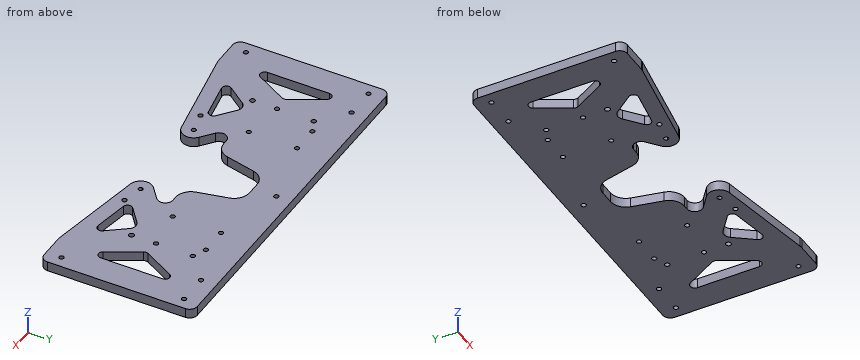
```python
from build123d import *

# Parameters (mm, degrees)
SKETCH1_W           = 233.2
SKETCH1_H           = 100
SKETCH1_R           = 1.55
BOSS_EXTRUDE1_DEPTH = 6.35
FILLET1_R           = 5
SKETCH2_R           = 1.55
CUT_EXTRUDE1_DEPTH  = 6.35
SKETCH3_W           = 10
SKETCH3_H           = 12.7
BOSS_EXTRUDE2_DEPTH = 6.35
FILLET2_R           = 5
FILLET3_R           = 10
FILLET4_R           = 2
FILLET5_R           = 20
FILLET6_R           = 5
CUT_EXTRUDE2_DEPTH  = 10
SKETCH5_W           = 120
SKETCH5_H           = 40
CUT_EXTRUDE4_DEPTH  = 10
SKETCH6_R           = 1.5
CUT_EXTRUDE5_DEPTH  = 10
FILLET7_R           = 10
SKETCH7_W           = 25
SKETCH7_H           = 35
CUT_EXTRUDE6_DEPTH  = 10
FILLET9_R           = 10
SKETCH8_R           = 1.5
CUT_EXTRUDE7_DEPTH  = 10
BOSS_EXTRUDE3_DEPTH = 6.35
FILLET10_R          = 5
BOSS_EXTRUDE4_DEPTH = 6.35
FILLET11_R          = 3
FILLET12_R          = 3
CUT_EXTRUDE8_DEPTH  = 10
FILLET13_R          = 3
CUT_EXTRUDE9_DEPTH  = 10
SKETCH13_R          = 1.55
CUT_EXTRUDE10_DEPTH = 10


with BuildPart() as part:
    # Sketch1 → Boss-Extrude1 (new body)
    with BuildSketch(Plane.XY):
        with Locations((116.6, -50)):
            Rectangle(SKETCH1_W, SKETCH1_H)
        with Locations((7.5, -10)):
            Circle(SKETCH1_R, mode=Mode.SUBTRACT)
        with Locations((225.7, -10)):
            Circle(SKETCH1_R, mode=Mode.SUBTRACT)
        with Locations((7.5, -90)):
            Circle(SKETCH1_R, mode=Mode.SUBTRACT)
        with Locations((225.7, -90)):
            Circle(SKETCH1_R, mode=Mode.SUBTRACT)
        with Locations((27.5, -10)):
            Circle(SKETCH1_R, mode=Mode.SUBTRACT)
        with Locations((205.7, -10)):
            Circle(SKETCH1_R, mode=Mode.SUBTRACT)
        with Locations((116.6, -10)):
            Circle(SKETCH1_R, mode=Mode.SUBTRACT)
    extrude(amount=BOSS_EXTRUDE1_DEPTH)

    # Fillet1
    fillet1_edges = [part.edges().sort_by_distance(p)[0] for p in [
        (233.2, -100, 3.175),
        (0, -100, 3.175),
        (0, 0, 3.175),
        (233.2, 0, 3.175),
    ]]
    fillet(fillet1_edges, radius=FILLET1_R)

    # Sketch2 → Cut-Extrude1 (cut)
    with BuildSketch(Plane.XY.offset(6.35)):
        with Locations((45, -25)):
            Circle(SKETCH2_R)
        with Locations((45, -49)):
            Circle(SKETCH2_R)
        with Locations(Location((188.2, -49, 0), (0, 0, 180))):
            Circle(SKETCH2_R)
        with Locations(Location((188.2, -25, 0), (0, 0, 180))):
            Circle(SKETCH2_R)
    extrude(amount=-CUT_EXTRUDE1_DEPTH, mode=Mode.SUBTRACT)

    # Sketch3 → Boss-Extrude2 (add)
    with BuildSketch(Plane.XY.offset(6.35)):
        with Locations((125.723568259, 6.35)):
            Rectangle(SKETCH3_W, SKETCH3_H)
        Polygon((120.723568259, 16.7), (120.723568259, 12.7), (130.723568259, 12.7), (130.723568259, 24.7), (85.723568259, 24.7), (85.723568259, 12.7), (95.723568259, 12.7), (95.723568259, 16.7), align=None)
        Polygon((130.723568259, 12.7), (130.723568259, 0), (152.313568259, 0), (130.723568259, 24.7), align=None)
    extrude(amount=-BOSS_EXTRUDE2_DEPTH)

    # Fillet2
    fillet2_edges = [part.edges().sort_by_distance(p)[0] for p in [
        (85.723568259, 12.7, 3.175),
    ]]
    fillet(fillet2_edges, radius=FILLET2_R)

    # Fillet3
    fillet3_edges = [part.edges().sort_by_distance(p)[0] for p in [
        (120.723568259, 0, 3.175),
    ]]
    fillet(fillet3_edges, radius=FILLET3_R)

    # Fillet4
    fillet4_edges = [part.edges().sort_by_distance(p)[0] for p in [
        (85.723568259, 24.7, 3.175),
    ]]
    fillet(fillet4_edges, radius=FILLET4_R)

    # Fillet5
    fillet5_edges = [part.edges().sort_by_distance(p)[0] for p in [
        (130.723568259, 24.7, 3.175),
        (152.313568259, 0, 3.175),
    ]]
    fillet(fillet5_edges, radius=FILLET5_R)

    # Fillet6
    fillet6_edges = [part.edges().sort_by_distance(p)[0] for p in [
        (120.723568259, 16.7, 3.175),
    ]]
    fillet(fillet6_edges, radius=FILLET6_R)

    # Sketch4 → Cut-Extrude2 (cut)
    with BuildSketch(Plane(origin=(0, 0, 0), x_dir=(-1, 0, 0), z_dir=(0, 0, -1))):
        with BuildLine():
            Line((-110.723568259, 0), (-161.395157905, 0))
            ThreePointArc((-161.395157905, 0), (-153.126132222, 1.789475179), (-146.33682816, 6.837678575))
            Line((-146.33682816, 6.837678575), (-136.700308357, 17.862321425))
            ThreePointArc((-136.700308357, 17.862321425), (-129.911004296, 22.910524821), (-121.641978613, 24.7))
            Line((-121.641978613, 24.7), (-87.723568259, 24.7))
            ThreePointArc((-87.723568259, 24.7), (-86.309354696, 24.114213562), (-85.723568259, 22.7))
            Line((-85.723568259, 22.7), (-85.723568259, 17.7))
            ThreePointArc((-85.723568259, 17.7), (-87.188034353, 14.164466094), (-90.723568259, 12.7))
            Line((-90.723568259, 12.7), (-95.723568259, 12.7))
            Line((-95.723568259, 12.7), (-95.723568259, 16.7))
            Line((-95.723568259, 16.7), (-115.723568259, 16.7))
            ThreePointArc((-115.723568259, 16.7), (-119.259102165, 15.235533906), (-120.723568259, 11.7))
            Line((-120.723568259, 11.7), (-120.723568259, 10))
            ThreePointArc((-120.723568259, 10), (-117.794636071, 2.928932188), (-110.723568259, 0))
        make_face()
    extrude(amount=-CUT_EXTRUDE2_DEPTH, mode=Mode.SUBTRACT)

    # Sketch5 → Cut-Extrude4 (cut)
    with BuildSketch(Plane.XY.offset(6.35)):
        Polygon((56.6, -100), (56.6, -60), (26.6, -100), align=None)
        with Locations((116.6, -80)):
            Rectangle(SKETCH5_W, SKETCH5_H)
        Polygon((206.6, -100), (176.6, -60), (176.6, -100), align=None)
    extrude(amount=-CUT_EXTRUDE4_DEPTH, mode=Mode.SUBTRACT)

    # Sketch6 → Cut-Extrude5 (cut)
    with BuildSketch(Plane.XY.offset(6.35)):
        with Locations((71.6, -21.25)):
            Circle(SKETCH6_R)
        with Locations((161.6, -21.25)):
            Circle(SKETCH6_R)
        with Locations((161.6, -52.75)):
            Circle(SKETCH6_R)
        with Locations((71.6, -52.75)):
            Circle(SKETCH6_R)
    extrude(amount=-CUT_EXTRUDE5_DEPTH, mode=Mode.SUBTRACT)

    # Fillet7
    fillet7_edges = [part.edges().sort_by_distance(p)[0] for p in [
        (206.6, -100, 3.175),
        (26.6, -100, 3.175),
        (56.6, -60, 3.175),
        (176.6, -60, 3.175),
    ]]
    fillet(fillet7_edges, radius=FILLET7_R)

    # Sketch7 → Cut-Extrude6 (cut)
    with BuildSketch(Plane.XY.offset(6.35)):
        Polygon((96.1, -60), (104.1, -60), (104.1, -25), align=None)
        Polygon((129.1, -25), (129.1, -60), (137.1, -60), align=None)
        with Locations((116.6, -42.5)):
            Rectangle(SKETCH7_W, SKETCH7_H)
    extrude(amount=-CUT_EXTRUDE6_DEPTH, mode=Mode.SUBTRACT)

    # Fillet9
    fillet9_edges = [part.edges().sort_by_distance(p)[0] for p in [
        (137.1, -60, 3.175),
        (96.1, -60, 3.175),
        (104.1, -25, 3.175),
        (129.1, -25, 3.175),
    ]]
    fillet(fillet9_edges, radius=FILLET9_R)

    # Sketch8 → Cut-Extrude7 (cut)
    with BuildSketch(Plane.XY.offset(6.35)):
        with Locations((53.6, -21.25)):
            Circle(SKETCH8_R)
        with Locations((179.6, -21.25)):
            Circle(SKETCH8_R)
    extrude(amount=-CUT_EXTRUDE7_DEPTH, mode=Mode.SUBTRACT)

    # Sketch9 → Boss-Extrude3 (add)
    with BuildSketch(Plane.XY.offset(6.35)):
        with BuildLine():
            Line((53.6, -64), (52.97582451, -64.832233986))
            Line((52.97582451, -64.832233986), (80.428117061, -87.022837132))
            ThreePointArc((80.428117061, -87.022837132), (90.975638571, -85.904897064), (89.857698503, -75.357375554))
            Line((89.857698503, -75.357375554), (70.858883385, -60))
            Line((70.858883385, -60), (61.6, -60))
            ThreePointArc((61.6, -60), (57.127864045, -61.05572809), (53.6, -64))
        make_face()
        with BuildLine():
            ThreePointArc((83.976361625, -80.247148199), (85.642998156, -79.775924736), (86.642907782, -81.190106343))
            ThreePointArc((86.642907782, -81.190106343), (84.642817409, -82.60428795), (83.976361625, -80.247148199))
        make_face(mode=Mode.SUBTRACT)
    boss_extrude3 = extrude(amount=-BOSS_EXTRUDE3_DEPTH)

    # Mirror1: Boss-Extrude3 across plane
    add(boss_extrude3.mirror(Plane.ZY.offset(-116.6)))

    # Fillet10
    fillet10_edges = [part.edges().sort_by_distance(p)[0] for p in [
        (52.97582451, -64.832233986, 3.175),
        (70.858883385, -60, 3.175),
        (180.22417549, -64.832233986, 3.175),
        (162.341116615, -60, 3.175),
    ]]
    fillet(fillet10_edges, radius=FILLET10_R)

    # Sketch10 → Boss-Extrude4 (add)
    with BuildSketch(Plane.XY.offset(6.35)):
        with BuildLine():
            ThreePointArc((29.6, -96), (26.844092638, -98.514663376), (23.358283237, -99.844208453))
            Line((23.358283237, -99.844208453), (86.46162021, -88.573262682))
            ThreePointArc((86.46162021, -88.573262682), (83.276282006, -88.454107183), (80.428117061, -87.022837132))
            Line((80.428117061, -87.022837132), (72.798322589, -80.855419933))
            Line((72.798322589, -80.855419933), (36.033483436, -87.422022085))
            Line((36.033483436, -87.422022085), (29.6, -96))
        make_face()
    boss_extrude4 = extrude(amount=-BOSS_EXTRUDE4_DEPTH)

    # Fillet11
    fillet11_edges = [part.edges().sort_by_distance(p)[0] for p in [
        (36.033483436, -87.422022085, 3.175),
        (72.798322589, -80.855419933, 3.175),
    ]]
    fillet(fillet11_edges, radius=FILLET11_R)

    # Mirror3: Boss-Extrude4 across plane
    add(boss_extrude4.mirror(Plane.ZY.offset(-116.6)))

    # Fillet12
    fillet12_edges = [part.edges().sort_by_distance(p)[0] for p in [
        (197.166516564, -87.422022085, 3.175),
        (160.401677411, -80.855419933, 3.175),
    ]]
    fillet(fillet12_edges, radius=FILLET12_R)

    # Sketch11 → Cut-Extrude8 (cut)
    with BuildSketch(Plane.XY.offset(6.35)):
        Polygon((35.5, -50), (18, -82), (18, -18), align=None)
        Polygon((215.2, -18), (215.2, -82), (197.7, -50), align=None)
    extrude(amount=-CUT_EXTRUDE8_DEPTH, mode=Mode.SUBTRACT)

    # Fillet13
    fillet13_edges = [part.edges().sort_by_distance(p)[0] for p in [
        (35.5, -50, 3.175),
        (18, -82, 3.175),
        (18, -18, 3.175),
        (215.2, -18, 3.175),
        (215.2, -82, 3.175),
        (197.7, -50, 3.175),
    ]]
    fillet(fillet13_edges, radius=FILLET13_R)

    # Sketch12 → Cut-Extrude9 (cut)
    with BuildSketch(Plane.XY.offset(6.35)):
        with BuildLine():
            ThreePointArc((186.5, -65), (188.2, -66.7), (189.9, -65))
            ThreePointArc((189.9, -65), (188.2, -63.3), (186.5, -65))
        make_face()
        with BuildLine():
            ThreePointArc((43.3, -65), (45, -66.7), (46.7, -65))
            ThreePointArc((46.7, -65), (45, -63.3), (43.3, -65))
        make_face()
    extrude(amount=-CUT_EXTRUDE9_DEPTH, mode=Mode.SUBTRACT)

    # Sketch13 → Cut-Extrude10 (cut)
    with BuildSketch(Plane.XY.offset(6.35)):
        with Locations((161.599999999, -84.25)):
            Circle(SKETCH13_R)
        with Locations((71.6, -84.25)):
            Circle(SKETCH13_R)
    extrude(amount=-CUT_EXTRUDE10_DEPTH, mode=Mode.SUBTRACT)


solid = part.part
```
Verification items for the finished model (mm, model axes). Coordinates: 2 decimals unless noted, no trailing zeros. Answer in a Markdown table with one row per item.
1) Section check A-A (z = 3). Give the number of separate pieces and of enclosed holes in the cut face, and give its area (3 significant figures).
The answers:
| item | result |
|---|---|
| separate pieces | 1 |
| enclosed holes | 27 |
| area | 17,200 mm2 |
2) Depth check by flat-ended pin: P1, Ø0.9, axis at x = 86, z = 4, coming from the -Y side; P2, Ø1, axis at x = 152.5, z = 2.5, coming from the -Y side; P3, Ø1.6, axis at x = 147.5, z = 3.5, coming from the -Y side. Enter the tip coordinate at first touch or a pass-through.
The answers:
| item | result |
|---|---|
| P1 | stops at y = -88.74 |
| P2 | stops at y = -89.69 |
| P3 | stops at y = -88.85 |
3) Scan lines: line 1 along Y through (x, z) = (225.7, 2.5); line 2 along X through (y, z) = (-40.5, 0.5); line 3 along X through (y, z) = (-34.5, 2.75). Record each from-to range of solid material in increasing order. Write a range as from..to.
The answers:
| item | result |
|---|---|
| line 1 | y = -100..-91.55, -88.45..-11.55, -8.45..0 |
| line 2 | x = 0..18, 30.3..100.56, 132.64..202.9, 215.2..233.2 |
| line 3 | x = 0..18, 27.02..101.93, 131.27..206.18, 215.2..233.2 |
